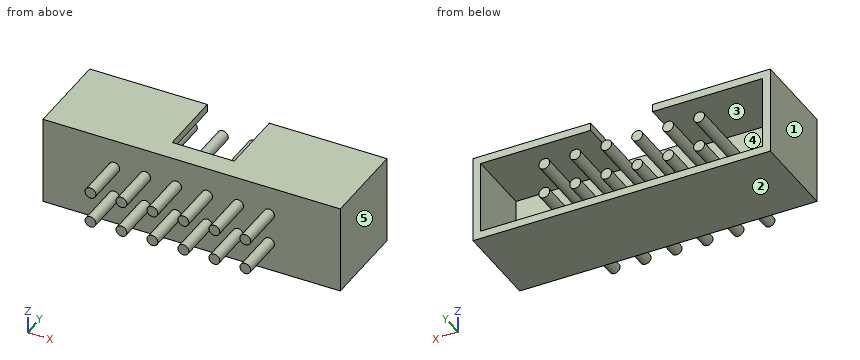
from build123d import *

# Parameters (mm, degrees)
SKETCH_1_W                  = 19.2
SKETCH_1_H                  = 5.7
EXTRUDE_1_DEPTH             = 5.7
SKETCH_2_W                  = 18.2
SKETCH_2_H                  = 4.7
CUT_EXTRUDE_1_DEPTH         = 4.3
CUT_EXTRUDE_2_REACH         = 7.7
SKETCH_3_W                  = 4
SKETCH_3_H                  = 4.3
SKETCH_4_R                  = 0.35
EXTRUDE_2_DEPTH             = 4.3
PATTERN_LINEAR_1_COUNT      = 6
PATTERN_LINEAR_1_PITCH      = 2
PATTERN_LINEAR_1_COUNT_DIR2 = 2
PATTERN_LINEAR_1_PITCH_DIR2 = 2


with BuildPart() as part:
    # 草图1 → 凸台-拉伸1 (new body)
    with BuildSketch(Plane(origin=(0, 0, 0), x_dir=(1, 0, 0), z_dir=(0, 1, 0))):
        with Locations((9.6, 2.85)):
            Rectangle(SKETCH_1_W, SKETCH_1_H)
    extrude(amount=EXTRUDE_1_DEPTH)

    # 草图2 → 切除-拉伸1 (cut)
    with BuildSketch(Plane(origin=(0, 5.7, 0), x_dir=(1, 0, 0), z_dir=(0, 1, 0))):
        with Locations((9.6, 2.85)):
            Rectangle(SKETCH_2_W, SKETCH_2_H)
    extrude(amount=-CUT_EXTRUDE_1_DEPTH, mode=Mode.SUBTRACT)

    # 草图3 → 切除-拉伸2 (cut, up to next)
    with BuildSketch(Plane.XY, mode=Mode.PRIVATE) as cut_extrude_2_sk1:
        with Locations((9.6, 3.55)):
            Rectangle(SKETCH_3_W, SKETCH_3_H)
    cut_extrude_2_tool1 = extrude(cut_extrude_2_sk1.sketch, amount=-CUT_EXTRUDE_2_REACH, mode=Mode.PRIVATE) & part.part
    add(cut_extrude_2_tool1.solids().sort_by_distance((9.6, 3.55, 0))[0], mode=Mode.SUBTRACT)

    # 草图4 → 凸台-拉伸2 (add, symmetric)
    with BuildSketch(Plane(origin=(0, 1.4, 0), x_dir=(1, 0, 0), z_dir=(0, 1, 0))):
        with Locations((4.6, 3.85)):
            Circle(SKETCH_4_R)
    extrude_2 = extrude(amount=EXTRUDE_2_DEPTH, both=True)

    # 阵列(线性)1: Extrude 2 6 × 2
    with Locations(*[(i * PATTERN_LINEAR_1_PITCH, 0, j * PATTERN_LINEAR_1_PITCH_DIR2) for i in range(PATTERN_LINEAR_1_COUNT) for j in range(PATTERN_LINEAR_1_COUNT_DIR2) if (i, j) != (0, 0)]):
        add(extrude_2)


solid = part.part
Input: part model. Units: mm. Frame: model coordinates. Face numbers are marked on the shaded views. A direction names the side the tool comes from. Round coordinates to 2 decimals unless told otherwise and drop trailing zeros. Loops run counter-clockwise (first coordinate to the right, second up) from the corner with the lowest first, then second, coordinate; pieces in that order, holes last. Notation, with made-up numbers: (17, -38) -> (67, -38) arc R19 ccw to (67, -19) -> close; hole circle Ø6 at (-8, -38). An arc over 180 degrees is marked (long way). Answer as a JSON object with one key per item and string values. Group by question number.
1) Section query C-C on x = 10.6. Output: boundary loops of the cut face in (y, z).
2) Draft query along Z for the marked faces 1, 2 and 3. Return one class per face: +Z half, -Z half, draft (parallel to the pull), parting line (faces both ways), or undercut.
3) Section query D-D on x = 4.6. Output: boundary loops of the cut face in (y, z), plus the area to 3 significant figures.
4) Ray query, L1, parallel to X at y = 3.5, z = -3; L2, parallel to Z at x = 16, y = 2.25; L3, parallel to Y at x = 18, z = -0.25. Return the intervals inside material, ascending.
5) Section query A-A on y = -2. State how many separate pieces and enclosed holes the cut face has, plus the area to 3 significant figures.
6) Section query B-B on z = -2.45. Output: boundary loops of the cut face in (x, y), plus the area to 3 significant figures.
7) Pin query (flat end, axial travel): pin 1 (1.5 mm diameter, centred on x = 5, y = -2, fed in from +Z); pin 2 (2.5 mm diameter, centred on x = 11.5, z = -3.5, fed in from +Y). Return the tip coordinate at first contact, or that it passes through.
8) Reachability of the marked faces 4 and 5 from +Z, -Z, +X, -X, +Y, -Y: full face, straight path, thin tool, end or side. Return the list, or none.
Reply:
{
 "1": {"outline": "(-2.9, -4.2) -> (0, -4.2) -> (0, -5.7) -> (5.7, -5.7) -> (5.7, -5.2) -> (1.4, -5.2) -> (1.4, -4.2) -> (5.7, -4.2) -> (5.7, -3.5) -> (1.4, -3.5) -> (1.4, -2.2) -> (5.7, -2.2) -> (5.7, -1.5) -> (1.4, -1.5) -> (1.4, 0) -> (0, 0) -> (0, -1.5) -> (-2.9, -1.5) -> (-2.9, -2.2) -> (0, -2.2) -> (0, -3.5) -> (-2.9, -3.5) -> close"},
 "2": {"face 1": "draft", "face 2": "-Z half", "face 3": "undercut"},
 "3": {"outline": "(-2.9, -4.2) -> (0, -4.2) -> (0, -5.7) -> (5.7, -5.7) -> (5.7, -5.2) -> (1.4, -5.2) -> (1.4, -4.2) -> (5.7, -4.2) -> (5.7, -3.5) -> (1.4, -3.5) -> (1.4, -2.2) -> (5.7, -2.2) -> (5.7, -1.5) -> (1.4, -1.5) -> (1.4, -0.5) -> (5.7, -0.5) -> (5.7, 0) -> (0, 0) -> (0, -1.5) -> (-2.9, -1.5) -> (-2.9, -2.2) -> (0, -2.2) -> (0, -3.5) -> (-2.9, -3.5) -> close", "area": "22.4 mm2"},
 "4": {"L1": "x = 0 to 0.5, 18.7 to 19.2", "L2": "z = -5.7 to -5.2, -0.5 to 0", "L3": "y = 0 to 5.7"},
 "5": {"separate pieces": "12", "enclosed holes": "0", "area": "4.62 mm2"},
 "6": {"outline": "(0, 0) -> (19.2, 0) -> (19.2, 5.7) -> (18.7, 5.7) -> (18.7, 1.4) -> (0.5, 1.4) -> (0.5, 5.7) -> (0, 5.7) -> close", "area": "31.2 mm2"},
 "7": {"pin 1": "stops at z = -1.5", "pin 2": "stops at y = 5.7"},
 "8": {"face 4": "+Y", "face 5": "+Z, -Z, +X, +Y, -Y"}
}
